Here's how the part is built. I have some questions about the finished solid (model axes, mm). Face numbers are marked on the shaded views. A direction names the side the tool comes from. Coordinates: 2 decimals unless noted, no trailing zeros. Loops run counter-clockwise (first coordinate to the right, second up) from the corner with the lowest first, then second, coordinate; pieces in that order, holes last. Notation, with made-up numbers: (-36.75, -30) -> (-16.75, -30) arc R26 cw to (-16.75, -6) -> close; hole circle Ø1 at (3.5, 42.25). An arc over 180 degrees is marked (long way). Answer as a JSON object with one key per item and string values. Group by question number.
1) I'm going to push flat-ended pins straight in: pin 1 (2 mm diameter, centred on x = -1, z = 7.5, fed in from +Y); pin 2 (3 mm diameter, centred on y = -1.5, z = 6, fed in from +X); pin 3 (1 mm diameter, centred on y = 1.5, z = 5.5, fed in from +X); pin 4 (1.2 mm diameter, centred on x = 0.5, z = 1, fed in from +Y). Where does each tip first touch, or does it pass through?
2) Which directions (+Z, -Z, +X, -X, +Y, -Y) give clear straight access to the entire face, cutting with the end or side of a thin tool? Please do the marked faces 1 and 2.
3) I want a section at A-A (x = 0). Write out the boundary of the cut face in (y, z) (3 decimals).
4) I need wall thicknesses on probe 1 along Z at (x, y) = (0.55, -0.8); probe 2 along Z at (x, y) = (-1.9, 1.15); probe 3 along Y at (x, z) = (0.4, 6). Which ranges of each line are inside material? Lowest first, please. Write a range as [from, to].
5) If we mould it in two halves opening along X, with no side actions, what happens to the marked faces 3, 4, 5 and 6? For each: +X half, -X half, draft (parallel to the pull), parting line (faces both ways), or undercut.
6) I want a section at B-B (z = 5.5). Write out the boundary of the cut face in (x, y).
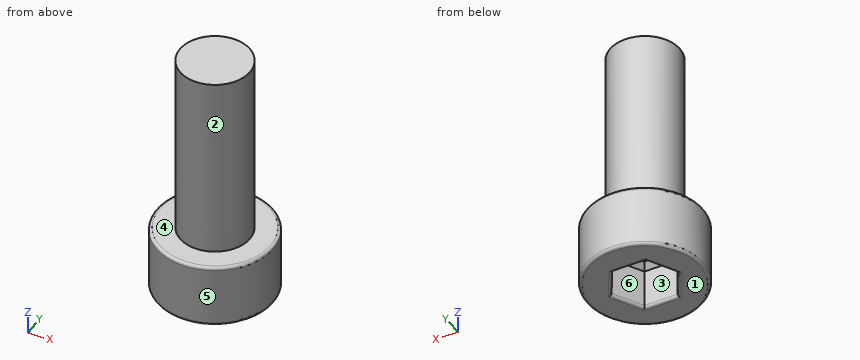
```python
from build123d import *

# Parameters (mm, degrees)
SKETCH1_R           = 2.5
BOSS_EXTRUDE1_DEPTH = 2.75
SKETCH2_R           = 1.5
BOSS_EXTRUDE2_DEPTH = 8
CUT_EXTRUDE1_DEPTH  = 2
CHAMFER1_SIZE       = 0.25
FILLET1_R           = 0.125


with BuildPart() as part:
    # Sketch1 → Boss-Extrude1 (new body)
    with BuildSketch(Plane.XY):
        Circle(SKETCH1_R)
    extrude(amount=BOSS_EXTRUDE1_DEPTH)

    # Sketch2 → Boss-Extrude2 (add)
    with BuildSketch(Plane.XY.offset(2.75)):
        Circle(SKETCH2_R)
    extrude(amount=BOSS_EXTRUDE2_DEPTH)

    # Sketch3 → Cut-Extrude1 (cut)
    with BuildSketch(Plane(origin=(0, 0, 0), x_dir=(-1, 0, 0), z_dir=(0, 0, -1))):
        Polygon((1.443375673, 0), (0.721687836, 1.25), (-0.721687836, 1.25), (-1.443375673, 0), (-0.721687836, -1.25), (0.721687836, -1.25), align=None)
    extrude(amount=-CUT_EXTRUDE1_DEPTH, mode=Mode.SUBTRACT)

    # Chamfer1
    chamfer1_edges = [part.edges().sort_by_distance(p)[0] for p in [
        (-1.082531755, -0.625, 2),
        (0, -1.25, 2),
        (1.082531755, -0.625, 2),
        (1.082531755, 0.625, 2),
        (0, 1.25, 2),
        (-1.082531755, 0.625, 2),
    ]]
    chamfer(chamfer1_edges, length=CHAMFER1_SIZE)

    # Fillet1
    fillet1_edges = [part.edges().sort_by_distance(p)[0] for p in [
        (-1.082531755, -0.625, 0),
        (-1.082531755, 0.625, 0),
        (0, 1.25, 0),
        (1.082531755, 0.625, 0),
        (1.082531755, -0.625, 0),
        (0, -1.25, 0),
        (-2.5, 0, 0),
        (-2.5, 0, 2.75),
    ]]
    fillet(fillet1_edges, radius=FILLET1_R)


solid = part.part
```
Determined:
{
 "1": {"pin 1": "y = 1.5", "pin 2": "x = 1.5", "pin 3": "x = 1.12", "pin 4": "y = 2.5"},
 "2": {"face 1": "-Z, +X, -X, +Y, -Y", "face 2": "+Z"},
 "3": {"outline": "(-2.5, 0.125) arc R0.125 ccw to (-2.375, 0) -> (-1.375, 0) arc R0.125 ccw to (-1.25, 0.125) -> (-1.25, 1.75) -> (-1, 2) -> (1, 2) -> (1.25, 1.75) -> (1.25, 0.125) arc R0.125 ccw to (1.375, 0) -> (2.375, 0) arc R0.125 ccw to (2.5, 0.125) -> (2.5, 2.625) arc R0.125 ccw to (2.375, 2.75) -> (1.5, 2.75) -> (1.5, 10.75) -> (-1.5, 10.75) -> (-1.5, 2.75) -> (-2.375, 2.75) arc R0.125 ccw to (-2.5, 2.625) -> close"},
 "4": {"probe 1": "[2, 10.75]", "probe 2": "[0, 2.75]", "probe 3": "[-1.45, 1.45]"},
 "5": {"face 3": "undercut", "face 4": "draft", "face 5": "parting line", "face 6": "undercut"},
 "6": {"outline": "circle Ø3 at (0, 0)"}
}
